Model file for the job. Use its own axes, mm. A direction names the side the tool comes from. Round coordinates to 2 decimals unless told otherwise and drop trailing zeros. Order: outer loops, then holes, each group sorted by start corner. A loop starts at its lowest first (then second) coordinate and runs counter-clockwise, first axis right, second up. Notation, with made-up numbers: (32, -39) - (60, -39) arc R21 cw to (60, -3) - close; hole circle Ø4 at (-32.75, -11.75). An arc over 180 degrees is marked (long way). Answer as CSV lines item,"result". Start each with the question number.
1. Wall check: line 1 along Y through (x, z) = (0, 2.75); line 2 along Y through (x, z) = (4, 2.9); line 3 along Y through (x, z) = (-12, 3.55). Give the ranges that are in metal, low to high. Write a range as [from, to].
2. Band-saw the part on D-D on y = 32.5. List the corners of the cut face in (x, z).
3. Pull direction Y, two halves, no side cores. Call faces 1 (the face through (12, 2, 5)), 2 (the face through (21.994, 0, 2)), 3 (the face through (9.5, 59.68, 2.46)), 4 (the face through (24.19, 4.32, 2.46)): released by +Y, released by -Y, zero draft, split by the parting line, or undercut.
4. Band-saw the part on A-A on y = -44. List the corners of the cut face in (x, z).
5. Band-saw the part on B-B on x = 0. List the corners of the cut face in (y, z), then the cut area to 3 significant figures.
6. 3-axis set-ups, long thin cutter, end or side, ignore diameter. For faces 5 (the face through (9.01, -58.34, 2.46)), 6 (the face through (21, 5.08, 2)): which of +Z, -Z, +X, -X, +Y, -Y reach the whole face in a straight line?
7. Band-saw the part on C-C on z = 3.85. List the corners of the cut face in (x, y).
8. Pin check, flat tips, straight feed: pin 1 Ø3 at (x, z) = (4, 3.5) entering from -Y; pin 2 Ø1.5 at (x, z) = (16.5, 1.5) entering from -Y; pin 3 Ø2 at (x, z) = (12.5, 2) entering from -Y; pin 4 Ø1 at (x, y) = (15, 50.5) entering from -Z. Stop position of each tip, or through.
```python
from build123d import *

# Parameters (mm, degrees)
F0_R     = 11
F1_DEPTH = 5


with BuildPart() as f1:
    # F0 (on Top) → F1 (new body)
    with BuildSketch(Plane.XY):
        with BuildLine():
            ThreePointArc((-5.328375, 46.857842), (7.061555, 45.914872), (13, 35))
            ThreePointArc((13, 35), (3.263036, 22.416177), (-11.361938, 28.682851))
            ThreePointArc((-11.361938, 28.682851), (-11.419195, 12.087231), (-22.790948, 0))
            ThreePointArc((-22.790948, 0), (-11.819872, -11.932631), (-11.032154, -28.123112))
            ThreePointArc((-11.032154, -28.123112), (3.576451, -22.50164), (13, -35))
            ThreePointArc((13, -35), (7.061555, -45.914872), (-5.328375, -46.857842))
            Line((-5.328375, -46.857842), (23.764569, -70.154617))
            Line((23.764569, -70.154617), (22.902545, -23.154617))
            ThreePointArc((22.902545, -23.154617), (17.870455, -14.524343), (15.235059, -4.888045))
            Line((15.235059, -4.888045), (26.443267, -4.888045))
            Line((26.443267, -4.888045), (21.993627, -3.388045))
            Line((21.993627, -3.388045), (21.993627, 3.58024))
            Line((21.993627, 3.58024), (26.443267, 5.08024))
            Line((26.443267, 5.08024), (15.172052, 5.08024))
            ThreePointArc((15.172052, 5.08024), (18.112091, 15.760837), (23.979004, 25.157556))
            Line((23.979004, 25.157556), (23.926978, 72.157556))
            Line((23.926978, 72.157556), (-5.328375, 46.857842))
        make_face()
        Circle(F0_R, mode=Mode.SUBTRACT)
        with BuildLine():
            ThreePointArc((-11.361938, 28.682851), (3.263036, 22.416177), (13, 35))
            ThreePointArc((13, 35), (7.061555, 45.914872), (-5.328375, 46.857842))
            ThreePointArc((-5.328375, 46.857842), (-11.941319, 40.13857), (-12.274144, 30.716847))
            ThreePointArc((-12.274144, 30.716847), (-11.792962, 29.711097), (-11.361938, 28.682851))
        make_face()
        with Locations((0, 35)):
            Circle(F0_R, mode=Mode.SUBTRACT)
        with BuildLine():
            ThreePointArc((13, -35), (3.576451, -22.50164), (-11.032154, -28.123112))
            ThreePointArc((-11.032154, -28.123112), (-12.436408, -38.786258), (-5.328375, -46.857842))
            ThreePointArc((-5.328375, -46.857842), (7.061555, -45.914872), (13, -35))
        make_face()
        with Locations((0, -35)):
            Circle(F0_R, mode=Mode.SUBTRACT)
    extrude(amount=F1_DEPTH)


solid = f1.part
```
Reply:
1,line 1,"y = [-51.12, -46], [-24, -11], [11, 24], [46, 51.47]"
1,line 2,"y = [-54.33, -45.25], [-24.75, -10.25], [10.25, 24.75], [45.25, 54.92]"
1,line 3,"y = [-40, -30], [-11.51, 10.76], [30.16, 40]"
2,outline,"(-12.76, 0) - (-10.71, 0) - (-10.71, 5) - (-12.76, 5) - close; (10.71, 0) - (23.97, 0) - (23.97, 5) - (10.71, 5) - close"
3,face 1,"zero draft"
3,face 2,"undercut"
3,face 3,"released by +Y"
3,face 4,"undercut"
4,outline,"(-9.38, 0) - (-6.32, 0) - (-6.32, 5) - (-9.38, 5) - close; (6.32, 0) - (23.28, 0) - (23.28, 5) - (6.32, 5) - close"
5,outline,"(-51.12, 0) - (-46, 0) - (-46, 5) - (-51.12, 5) - close; (-24, 0) - (-11, 0) - (-11, 5) - (-24, 5) - close; (11, 0) - (24, 0) - (24, 5) - (11, 5) - close; (46, 0) - (51.47, 0) - (51.47, 5) - (46, 5) - close"
5,area,"183 mm2"
6,face 5,"+Z, -Z, -X, -Y"
6,face 6,"+Z, -Z, +X"
7,outline,"(-22.79, 0) arc R23.81 cw to (-11.03, -28.12) arc R13 ccw to (-5.33, -46.86) - (23.76, -70.15) - (22.9, -23.15) arc R38.4 cw to (15.24, -4.89) - (26.44, -4.89) - (21.99, -3.39) - (21.99, 3.58) - (26.44, 5.08) - (15.17, 5.08) arc R38.4 cw to (23.98, 25.16) - (23.93, 72.16) - (-5.33, 46.86) arc R13 ccw to (-12.27, 30.72) arc R22.61 cw to (-11.36, 28.68) arc R22.61 cw to start; hole circle Ø22 at (0, -35); hole circle Ø22 at (0, 0); hole circle Ø22 at (0, 35)"
8,pin 1,"stops at y = -55.53"
8,pin 2,"stops at y = -64.94"
8,pin 3,"stops at y = -61.94"
8,pin 4,"stops at z = 0"
